Check sheet for the modelled part. Datum: model origin and axes. Units: mm. Round coordinates to 2 decimals unless told otherwise and drop trailing zeros. Order: outer loops, then holes, each group sorted by start corner. A loop starts at its lowest first (then second) coordinate and runs counter-clockwise, first axis right, second up.
(1) Sectioned sample at B-B, the plane z = 8.5. Enter the section's corners in (x, y), and give its area (3 significant figures).
(2) Thickness scan on probe 1 along Y at (x, z) = (0, 4); probe 2 along X at (y, z) = (3, 9.75); probe 3 along Y at (x, z) = (10, 6.5). Record the ranges inside material, lowest first.
(3) Sectioned sample at C-C, the plane y = 8. Enter the section's corners in (x, z), and give its area (3 significant figures).
(4) Sectioned sample at D-D, the plane x = -15. Enter the section's corners in (y, z).
(5) Depth check by flat-ended pin: pin 1 (2 mm diameter, centred on y = -0.5, z = 3.5, fed in from -X); pin 2 (6 mm diameter, centred on y = -6.5, z = 7.5, fed in from -X); pin 3 (1.5 mm diameter, centred on x = -12.5, z = 5.5, fed in from -Y). Enter the tip coordinate at first touch or a pass-through.
(6) Mould release check, pull along Y, two halves, no side actions. Record for faces 1 (the flat face through (13.8, -8.1, 4.9)), 2 (the cylindrical face through (11.923, -3.755, 4.93)), 3 (the flat face through (13.92, 7.89, 4.93)), 4 (the flat face through (12.2, 3.6, 10)): released by +Y, released by -Y, zero draft, split by the parting line, or undercut.
(7) Sectioned sample at A-A, the plane x = 0. Enter the section's corners in (y, z), and give its area (3 significant figures).
Solid Edge part; units mm, degrees
sketch "Sketch1" plane through (0, 0, 0) normal (0, 0, 1) x (1, 0, 0)
  circle A0 centre (0, 0) radius 12.5
  line L0 (-9.2376, 16) -> (-18.4752, 0)
  line L1 (-18.4752, 0) -> (-9.2376, -16)
  line L2 (-9.2376, -16) -> (9.2376, -16)
  line L3 (9.2376, -16) -> (18.4752, 0)
  line L4 (18.4752, 0) -> (9.2376, 16)
  line L5 (9.2376, 16) -> (-9.2376, 16)
extrude "Protrusion1" add sketch "Sketch1" along normal blind 10
Derived:
1. outline: (-18.48, 0) - (-9.24, -16) - (9.24, -16) - (18.48, 0) - (9.24, 16) - (-9.24, 16) - close; hole circle Ø25 at (0, 0)
1. area: 396 mm2
2. probe 1: y = -16 to -12.5, 12.5 to 16
2. probe 2: x = -16.74 to -12.13, 12.13 to 16.74
2. probe 3: y = -14.68 to -7.5, 7.5 to 14.68
3. outline: (-13.86, 0) - (-9.6, 0) - (-9.6, 10) - (-13.86, 10) - close; (9.6, 0) - (13.86, 0) - (13.86, 10) - (9.6, 10) - close
3. area: 85.0 mm2
4. outline: (-6.02, 0) - (6.02, 0) - (6.02, 10) - (-6.02, 10) - close
5. pin 1: stops at x = -18.48
5. pin 2: stops at x = -16.45
5. pin 3: stops at y = -11.65
6. face 1: released by -Y
6. face 2: undercut
6. face 3: released by +Y
6. face 4: zero draft
7. outline: (-16, 0) - (-12.5, 0) - (-12.5, 10) - (-16, 10) - close; (12.5, 0) - (16, 0) - (16, 10) - (12.5, 10) - close
7. area: 70.0 mm2
